Input: part model. Units: mm. Frame: model coordinates. A direction names the side the tool comes from. Coordinates: 2 decimals unless noted, no trailing zeros. Loops run counter-clockwise (first coordinate to the right, second up) from the corner with the lowest first, then second, coordinate; pieces in that order, holes last. Notation, with made-up numbers: (65.25, -28.75) - (98.25, -28.75) arc R20 cw to (98.25, -1.75) - close; hole circle Ø7 at (26, -36.5). An arc over 180 degrees is marked (long way). Use a Markdown table: item, result. Add a question column.
1. Access query for faces 4 (the face through (0.1, 3.9, 56.3)), 5 (the face through (0, 19, -36)), 6 (the face through (-1.5, 15.2, -30)), 7 (the face through (16, 5.368, -36)). Directions: +Z, -Z, +X, -X, +Y, -Y. A direction counts if a zero-diameter tool reaches every point of the face in a straight line with its end or side. Return the directions, or none.
2. Ray query, L1, parallel to Z at x = -9.5, y = 13.5; L2, parallel to X at y = 10.5, z = -41; L3, parallel to Y at x = -5.5, z = -35. Return the intervals inside material, ascending. Write a range as [from, to].
3. Draft query along Z for faces 1 (the face through (0, 8, 41.5)), 2 (the face through (-16, 5.368, 36)), 3 (the face through (0, 15, 0)). Return one class per face: released by +Z, released by -Z, zero draft, split by the parting line, or undercut.
4. Section query B-B on z = 36. Return the cut outline in (x, y) (1 decimal).
5. Section query D-D on z = -49.5. Return the cut outline in (x, y), then the cut area to 3 significant figures.
6. Section query A-A on x = 0. Return the cut outline in (y, z).
7. Section query C-C on y = 10.5. Return the cut outline in (x, z), then the cut area to 3 significant figures.
8. Contact query for flat-ended pins moving along their axis: P1, Ø5.5, axis at x = 5, y = 7, coming from the +Z side; P2, Ø1.8, axis at x = 17, z = -36.5, coming from the +Y side; P3, Ø3, axis at x = 16, z = 36.5, coming from the +Y side. Output: stop coordinate, or through.
```python
from build123d import *

# Parameters (mm, degrees)
F1_DEPTH = 41.5
F3_DEPTH = 30
F5_DEPTH = 30
F7_DEPTH = 113.001
F9_DEPTH = 30


with BuildPart() as f1:
    # F0 (on Top) → F1 (new body, symmetric)
    with BuildSketch(Plane.XY):
        with BuildLine():
            Line((-19, 0), (19, 0))
            ThreePointArc((19, 0), (0, 19), (-19, 0))
        make_face()
    extrude(amount=F1_DEPTH, both=True)

    # F2 (on face) → F3 (join)
    with BuildSketch(Plane.XY.offset(41.5)):
        with BuildLine():
            Line((-3.9, 0), (3.9, 0))
            ThreePointArc((3.9, 0), (0, 3.9), (-3.9, 0))
        make_face()
    extrude(amount=F3_DEPTH)

    # F4 (on face) → F5 (join)
    with BuildSketch(Plane(origin=(0, 0, -41.5), x_dir=(1, 0, 0), z_dir=(0, 0, -1))):
        with BuildLine():
            Line((3.9, 0), (-3.9, 0))
            ThreePointArc((-3.9, 0), (0, -3.9), (3.9, 0))
        make_face()
    extrude(amount=F5_DEPTH)

    # F6 (on face) → F7 (cut, through all)
    with BuildSketch(Plane.XY.offset(41.5)):
        with BuildLine():
            Line((-14.568067, 5.368078), (-14.568067, 12.197189))
            ThreePointArc((-14.568067, 12.197189), (-16.748743, 8.971042), (-18.225909, 5.368078))
            Line((-18.225909, 5.368078), (-14.568067, 5.368078))
        make_face()
        with BuildLine():
            Line((-4.264999, 14.724803), (-4.264999, 18.515123))
            ThreePointArc((-4.264999, 18.515123), (-8.354055, 17.06487), (-12.007505, 14.724803))
            Line((-12.007505, 14.724803), (-4.264999, 14.724803))
        make_face()
        with BuildLine():
            ThreePointArc((12.007505, 14.724803), (8.354055, 17.06487), (4.264999, 18.515123))
            Line((4.264999, 18.515123), (4.264999, 14.724803))
            Line((4.264999, 14.724803), (12.007505, 14.724803))
        make_face()
        with BuildLine():
            ThreePointArc((18.225909, 5.368078), (16.748743, 8.971042), (14.568067, 12.197189))
            Line((14.568067, 12.197189), (14.568067, 5.368078))
            Line((14.568067, 5.368078), (18.225909, 5.368078))
        make_face()
    extrude(amount=-F7_DEPTH, mode=Mode.SUBTRACT)

    # F8 (on Top) → F9 (cut, symmetric)
    with BuildSketch(Plane.XY):
        with BuildLine():
            Line((15, 0), (22.459483, 0))
            ThreePointArc((22.459483, 0), (0, 22.459483), (-22.459483, 0))
            Line((-22.459483, 0), (-15, 0))
            ThreePointArc((-15, 0), (0, 15), (15, 0))
        make_face()
    extrude(amount=F9_DEPTH, both=True, mode=Mode.SUBTRACT)


solid = f1.part
```
Resolved:
| question | item | result |
|---|---|---|
| 1 | face 4 | +Z, +Y |
| 1 | face 5 | +Z, -Z, +Y |
| 1 | face 6 | +Y |
| 1 | face 7 | +Z, -Z, +X, +Y |
| 2 | L1 | [-41.5, -30], [30, 41.5] |
| 2 | L2 | [-14.57, 14.57] |
| 2 | L3 | [0, 14.72] |
| 3 | face 1 | released by +Z |
| 3 | face 2 | zero draft |
| 3 | face 3 | undercut |
| 4 | outline | (-19, 0) - (19, 0) arc R19 ccw to (18.2, 5.4) - (14.6, 5.4) - (14.6, 12.2) arc R19 ccw to (12, 14.7) - (4.3, 14.7) - (4.3, 18.5) arc R19 ccw to (-4.3, 18.5) - (-4.3, 14.7) - (-12, 14.7) arc R19 ccw to (-14.6, 12.2) - (-14.6, 5.4) - (-18.2, 5.4) arc R19 ccw to start |
| 5 | outline | (-3.9, 0) - (3.9, 0) arc R3.9 ccw to start |
| 5 | area | 23.9 mm² |
| 6 | outline | (0, -71.5) - (3.9, -71.5) - (3.9, -41.5) - (19, -41.5) - (19, -30) - (15, -30) - (15, 30) - (19, 30) - (19, 41.5) - (3.9, 41.5) - (3.9, 71.5) - (0, 71.5) - close |
| 7 | outline | (-14.57, -41.5) - (14.57, -41.5) - (14.57, -30) - (10.71, -30) - (10.71, 30) - (14.57, 30) - (14.57, 41.5) - (-14.57, 41.5) - (-14.57, 30) - (-10.71, 30) - (-10.71, -30) - (-14.57, -30) - close |
| 7 | area | 1,960 mm² |
| 8 | P1 | z = 41.5 |
| 8 | P2 | y = 5.37 |
| 8 | P3 | y = 12.28 |
